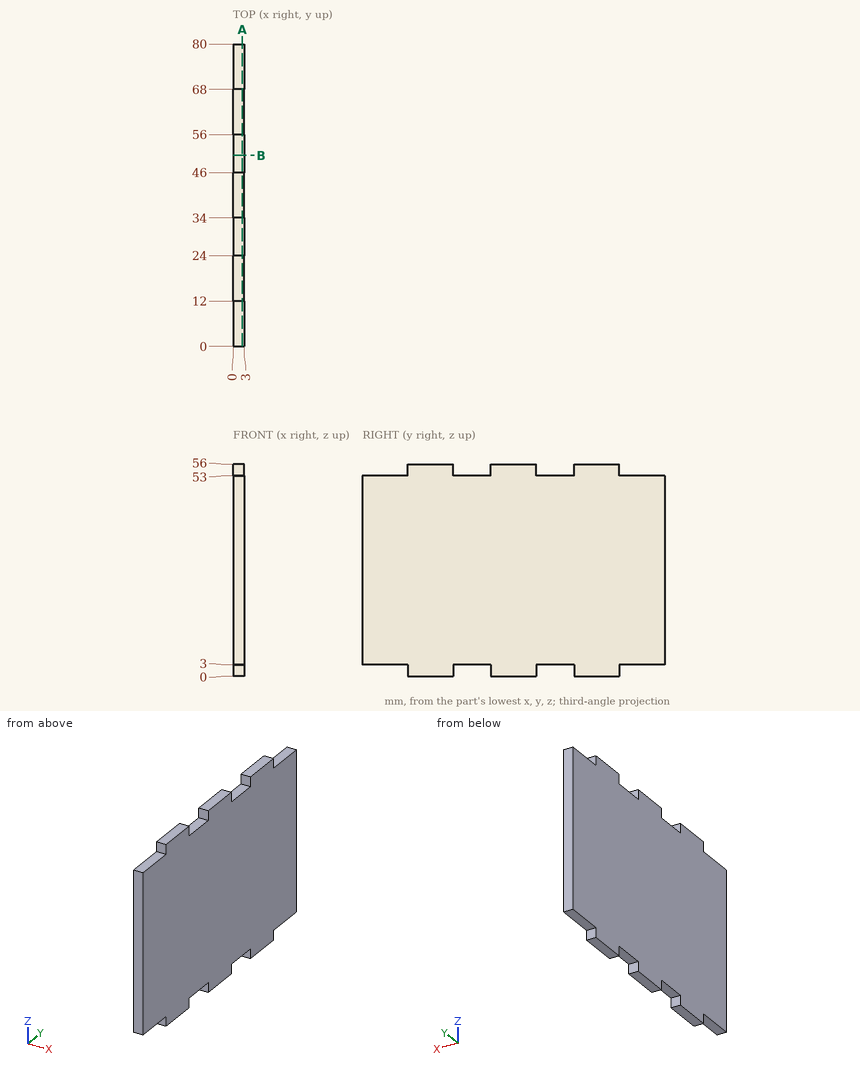
Verification items for this drawing (mm, ordinates from the low corner). Coordinates: 2 decimals unless noted, no trailing zeros. Order: outer loops, then holes, each group sorted by start corner. A loop starts at its lowest first (then second) coordinate and runs counter-clockwise, first axis right, second up. Notation, with made-up numbers: (67.25, -25.5) - (79.25, -25.5) arc R11 cw to (79.25, -17.5) - close; hole circle Ø9 at (-8, -29.75). An arc over 180 degrees is marked (long way). Answer as a JSON object with one key per item and string values. Group by question number.
Item 1: Depth check by flat-ended pin: pin 1 Ø0.9 at (x, z) = (1, 54.5) entering from +Y; pin 2 Ø0.9 at (x, y) = (1.5, 30.5) entering from -Z; pin 3 Ø1.5 at (x, y) = (2, 31.5) entering from +Z. Enter the tip coordinate at first touch or a pass-through.
Item 2: Sectioned sample at B-B, the plane y = 50.5. Record the cut outline in (x, z), and give its area (3 significant figures).
Item 3: Sectioned sample at A-A, the plane x = 2.45. Record the cut outline in (y, z).
Item 4: Scan line: probe 1 along Z at (x, y) = (0.6, 5). Record every from-to range of solid material in increasing order.
Resolved:
{
 "1": {"pin 1": "y = 68", "pin 2": "z = 3", "pin 3": "z = 53"},
 "2": {"outline": "(0, 3) - (3, 3) - (3, 53) - (0, 53) - close", "area": "150 mm^2"},
 "3": {"outline": "(0, 3) - (12, 3) - (12, 0) - (24, 0) - (24, 3) - (34, 3) - (34, 0) - (46, 0) - (46, 3) - (56, 3) - (56, 0) - (68, 0) - (68, 3) - (80, 3) - (80, 53) - (68, 53) - (68, 56) - (56, 56) - (56, 53) - (46, 53) - (46, 56) - (34, 56) - (34, 53) - (24, 53) - (24, 56) - (12, 56) - (12, 53) - (0, 53) - close"},
 "4": {"probe 1": "3 to 53"}
}
